Input: dimensioned drawing with shaded views. Units: mm. Origin: part minimum x, y, z. A direction names the side the tool comes from. Give positions to 0.01 mm unless a question says otherwise; leave off trailing zeros. Loops run counter-clockwise (first coordinate to the right, second up) from the corner with the lowest first, then second, coordinate; pieces in that order, holes last. Notation, with made-up numbers: (-27, 74.25) -> (-2, 74.25) arc R28 ccw to (-2, 99.25) -> close; hole circle Ø7 at (33, 22). An arc over 180 degrees is marked (long way). Answer in a Markdown table with one row per item. Add a question column.
1) Line query: line 1 (X direction, y = 2.7, z = 4); line 2 (Z direction, x = 4, y = 2.7); line 3 (X direction, y = 1.85, z = 28). Output: solid intervals per line, ascending. Write a range as from..to.
2) Draft query along X for the marked faces 1 and 2. Return one class per face: +X half, -X half, draft (parallel to the pull), parting line (faces both ways), or undercut.
3) Section query B-B (x = 4). Return the cut outline in (y, z) (3 decimals).
4) Section query D-D (z = 17.75). Return the cut outline in (x, y), plus the area to 3 significant figures.
5) First-contact query: P1, Ø0.8, axis at x = 57, y = 0.5, coming from the -Z side; P2, Ø1.5, axis at x = 37, y = 1.5, coming from the -Z side; P3, Ø4, axis at x = 8.5, z = 26, coming from the -Y side; P4, Ø0.8, axis at x = 22.5, y = 1.5, coming from the +Z side. Flat tips, straight axial feed; report the tip coordinate or a pass-through.
6) Access query for the marked faces 3 and 4. Directions: +Z, -Z, +X, -X, +Y, -Y. A direction counts if a zero-diameter tool reaches every point of the face in a straight line with its end or side. Return the directions, or none.
7) Section query C-C (x = 18). Return the cut outline in (y, z).
8) Section query A-A (z = 4). Return the cut outline in (x, y) (3 decimals).
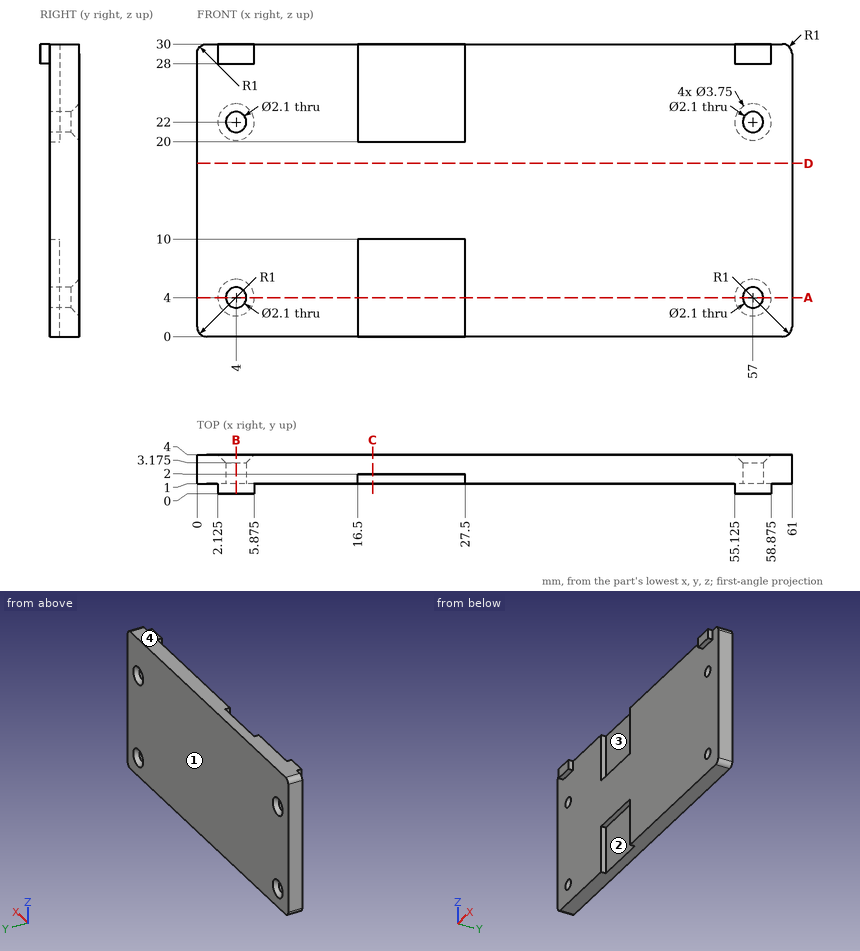
Evaluation:
| question | item | result |
|---|---|---|
| 1 | line 1 | 0..2.95, 5.05..55.95, 58.05..61 |
| 1 | line 2 | 0..2.95, 5.05..20.95, 23.05..30 |
| 1 | line 3 | 0..16.5, 27.5..61 |
| 2 | face 1 | draft |
| 2 | face 2 | undercut |
| 3 | outline | (0, 28) -> (1, 28) -> (1, 23.05) -> (3.175, 23.05) -> (4, 23.875) -> (4, 30) -> (0, 30) -> close; (1, 0) -> (4, 0) -> (4, 2.125) -> (3.175, 2.95) -> (1, 2.95) -> close; (1, 5.05) -> (3.175, 5.05) -> (4, 5.875) -> (4, 20.125) -> (3.175, 20.95) -> (1, 20.95) -> close |
| 4 | outline | (0, 1) -> (61, 1) -> (61, 4) -> (0, 4) -> close |
| 4 | area | 183 mm² |
| 5 | P1 | z = 28 |
| 5 | P2 | z = 0 |
| 5 | P3 | y = 1 |
| 5 | P4 | z = 20 |
| 6 | face 3 | +Z, -Y |
| 6 | face 4 | +Z, +X, -X, +Y, -Y |
| 7 | outline | (1, 10) -> (2, 10) -> (2, 0) -> (4, 0) -> (4, 30) -> (2, 30) -> (2, 20) -> (1, 20) -> close |
| 8 | outline | (0, 1) -> (2.95, 1) -> (2.95, 3.175) -> (2.125, 4) -> (0, 4) -> close; (5.05, 1) -> (16.5, 1) -> (16.5, 2) -> (27.5, 2) -> (27.5, 1) -> (55.95, 1) -> (55.95, 3.175) -> (55.125, 4) -> (5.875, 4) -> (5.05, 3.175) -> close; (58.05, 1) -> (61, 1) -> (61, 4) -> (58.875, 4) -> (58.05, 3.175) -> close |
